Check sheet for the drawn part. Datum: minimum x, y, z corner. Units: mm. A direction names the side the tool comes from. Coordinates: 2 decimals unless noted, no trailing zeros. Order: outer loops, then holes, each group sorted by start corner. A loop starts at its lowest first (then second) coordinate and runs counter-clockwise, first axis right, second up. Notation, with made-up numbers: (14, -0.75) - (49, -0.75) arc R14 cw to (49, 13.25) - close; hole circle Ø7 at (60, 45). An arc over 180 degrees is marked (long way). One line per item, written item: value. Start each with the question number.
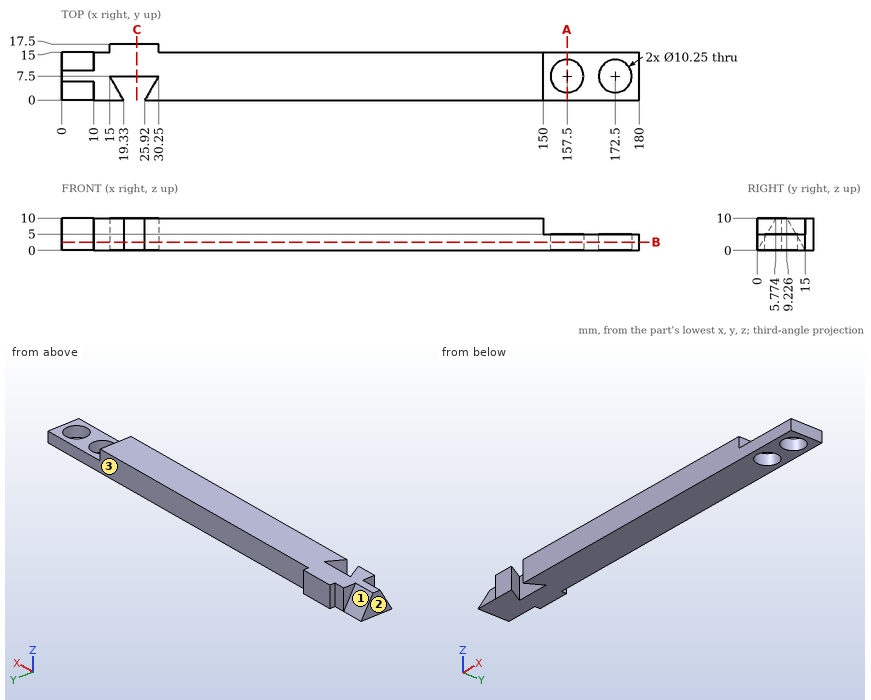
Q1. Cross-section at A-A, the plane x = 157.5. Enter the section's corners in (y, z) (1 decimal).
Q2. Cross-section at C-C, the plane x = 23.5. Enter the section's corners in (y, z), and give its area (3 significant figures).
Q3. Gauge pin test, flat ends, axial feed: P1, Ø5, axis at x = 136, z = 4.5, coming from the +Y side; P2, Ø9, axis at x = 172.5, y = 7.5, coming from the -Z side; P3, Ø7.5, axis at x = 165, y = 6.5, coming from the +Z side; P4, Ø3, axis at y = 15.5, z = 7.5, coming from the -X side. Record the tip position at first contact, or that the pin passes through.
Q4. Set-up check for the marked faces 1, 2 and 3: record each of +Z, -Z, +X, -X, +Y, -Y from which the full face is reachable in a straight line by a thin tool's end or side.
Q5. Cross-section at B-B, the plane z = 2.5. Count the separate pieces of the cut face and the enclosed holes in it, and give its area (3 significant figures).
Q6. Material ranges on probe 1 along X at (y, z) = (8, 1.25); probe 2 along Y at (x, z) = (157.5, 3.35) (1 decimal); probe 3 along Y at (x, z) = (111.5, 8.5), recorded low to high.
Check result:
1. outline: (0, 0) - (2.4, 0) - (2.4, 5) - (0, 5) - close; (12.6, 0) - (15, 0) - (15, 5) - (12.6, 5) - close
2. outline: (7.5, 0) - (17.5, 0) - (17.5, 10) - (7.5, 10) - close
2. area: 100 mm2
3. P1: stops at y = 15
3. P2: passes through
3. P3: stops at z = 5
3. P4: stops at x = 10
4. face 1: +Z, -X, +Y
4. face 2: +Z, -Z, -X, +Y, -Y
4. face 3: +Z, -Z, +X, +Y
5. separate pieces: 1
5. enclosed holes: 2
5. area: 2,460 mm2
6. probe 1: x = 0 to 152.4, 162.6 to 167.4, 177.6 to 180
6. probe 2: y = 0 to 2.4, 12.6 to 15
6. probe 3: y = 0 to 15
